Work out the finished part from the listing and answer in its coordinate system (mm). A direction names the side the tool comes from. Give positions to 0.01 mm unless a question says otherwise; leave off trailing zeros. Loops run counter-clockwise (first coordinate to the right, second up) from the corner with the lowest first, then second, coordinate; pieces in that order, holes last.
from build123d import *

# Parameters (mm, degrees)
SKETCH1_R           = 8.5
SKETCH1_R_2         = 2.5
BOSS_EXTRUDE1_DEPTH = 23
SKETCH3_W           = 5.8
SKETCH3_H           = 2.8
CUT_EXTRUDE2_DEPTH  = 8
SKETCH7_W           = 5.8
SKETCH7_H           = 2.8
CUT_EXTRUDE5_DEPTH  = 8
SKETCH4_R           = 1.65
CUT_EXTRUDE3_DEPTH  = 9.5


with BuildPart() as part:
    # Sketch1 → Boss-Extrude1 (new body)
    with BuildSketch(Plane(origin=(0, 0, 0), x_dir=(1, 0, 0), z_dir=(0, 1, 0))):
        Circle(SKETCH1_R)
        Circle(SKETCH1_R_2, mode=Mode.SUBTRACT)
    extrude(amount=BOSS_EXTRUDE1_DEPTH)

    # Sketch3 → Cut-Extrude2 (cut)
    with BuildSketch(Plane(origin=(0, 23, 0), x_dir=(1, 0, 0), z_dir=(0, 1, 0))):
        with Locations((0, 5)):
            Rectangle(SKETCH3_W, SKETCH3_H)
    cut_extrude2 = extrude(amount=-CUT_EXTRUDE2_DEPTH, mode=Mode.SUBTRACT)

    # Sketch7 → Cut-Extrude5 (cut)
    with BuildSketch(Plane.XZ):
        with Locations((0, -5.5)):
            Rectangle(SKETCH7_W, SKETCH7_H)
    extrude(amount=-CUT_EXTRUDE5_DEPTH, mode=Mode.SUBTRACT)

    # Sketch4 → Cut-Extrude3 (cut, through all)
    with BuildSketch(Plane.XY):
        with Locations((0, 19)):
            Circle(SKETCH4_R)
        with Locations((0, 4)):
            Circle(SKETCH4_R)
    extrude(amount=-CUT_EXTRUDE3_DEPTH, mode=Mode.SUBTRACT)

    # Mirror1: Cut-Extrude2 across plane
    add(cut_extrude2.mirror(Plane.XY), mode=Mode.SUBTRACT)


solid = part.part
Item 1: Determine the mould class of faces 1 (the face through (0, 19, 6.4)), 2 (the face through (-0.215, 20.636, -2.918)), 3 (the face through (0, 15, -5)) for opening direction Y: released by +Y, released by -Y, zero draft, split by the parting line, or undercut.
Item 2: Flat-ended cylindrical pins translate along their axes: pin 1 Ø0.8 at (y, z) = (4, -5) entering from -X; pin 2 Ø3 at (x, y) = (0, 19) entering from -Z; pin 3 Ø1.4 at (y, z) = (20, 5.5) entering from +X (3 decimals). Find the tip coordinate at first contact, or state that the pin passes through.
Item 3: Find section B-B, the plane y = 19. Write down the section's boundary in (x, z).
Item 4: Find section D-D, the plane y = 7.5. Write down the section's boundary in (x, z).
Item 5: Find section C-C, the plane x = -2. Write down the section's boundary in (y, z), plus the area to 3 significant figures.
Item 6: For faces 4 (the face through (0, 8, -5)), 5 (the face through (2, 0, 2)), 6 (the face through (-2.9, 19, -5)), 7 (the face through (-1.84, 11.34, 8.3)), 8 (the face through (-0.215, 5.636, -7.691)), determine the directions among +Z, -Z, +X, -X, +Y, -Y from which every point of the face is accessible in a straight line to the end or side of a thin tool.
Item 7: Find section A-A, the plane z = 0. Write down the section's boundary in (x, y).
Item 8: Consider line 1 (Y direction, x = 0, z = -8.1); line 2 (Z direction, x = 0, y = 9.25). Determine where each line is inside the solid, lowest interval first.
Ans:
1. face 1: zero draft
1. face 2: undercut
1. face 3: released by +Y
2. pin 1: stops at x = -7.15
2. pin 2: stops at z = 2
2. pin 3: stops at x = 7.015
3. outline: (-2.9, -6.4) - (-2.9, -3.6) - (-1.65, -3.6) - (-1.65, -1.88) arc R2.5 cw (long way) to (1.65, -1.88) - (1.65, -3.6) - (2.9, -3.6) - (2.9, -6.4) - (1.65, -6.4) - (1.65, -8.34) arc R8.5 ccw (long way) to (-1.65, -8.34) - (-1.65, -6.4) - close; hole (-2.9, 3.6) - (2.9, 3.6) - (2.9, 6.4) - (-2.9, 6.4) - close
4. outline: circle Ø17 at (0, 0); hole (-2.9, -6.9) - (2.9, -6.9) - (2.9, -4.1) - (-2.9, -4.1) - close; hole circle Ø5 at (0, 0)
5. outline: (0, -8.26) - (23, -8.26) - (23, -6.4) - (15, -6.4) - (15, -3.6) - (23, -3.6) - (23, -1.5) - (0, -1.5) - (0, -4.1) - (8, -4.1) - (8, -6.9) - (0, -6.9) - close; (0, 1.5) - (23, 1.5) - (23, 3.6) - (15, 3.6) - (15, 6.4) - (23, 6.4) - (23, 8.26) - (0, 8.26) - close
5. area: 244 mm2
6. face 4: -Y
6. face 5: +Z, -Z, +X, -X, -Y
6. face 6: +Y
6. face 7: +Y, -Y
6. face 8: -Z
7. outline: (-8.5, 0) - (-2.5, 0) - (-2.5, 23) - (-8.5, 23) - close; (2.5, 0) - (8.5, 0) - (8.5, 23) - (2.5, 23) - close
8. line 1: y = 0 to 2.35, 5.65 to 17.35, 20.65 to 23
8. line 2: z = -8.5 to -2.5, 2.5 to 8.5
